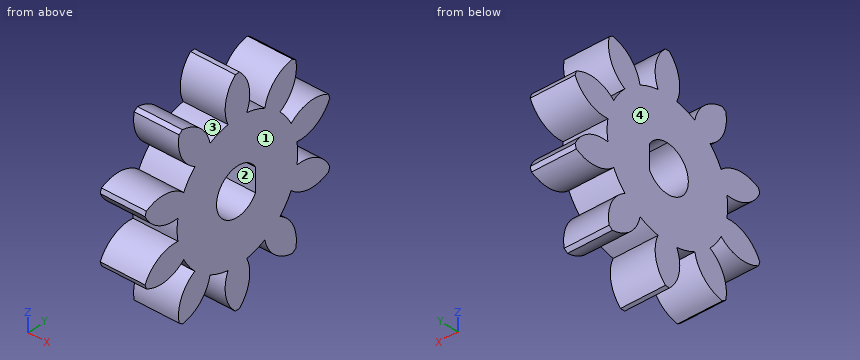
```python
from build123d import *

# Parameters (mm, degrees)
BASPROSKE_W        = 5
BASPROSKE_H        = 12
TOOTHCUT_DEPTH     = 18.691806013
TEETHCUTS_COUNT    = 10
TEETHCUTS_ANGLE    = 324
BORSKE_R           = 0.5
BORE_DEPTH         = 50.0000508
SKETCH2_R          = 0.5
CUT_EXTRUDE1_DEPTH = 10


with BuildPart() as part:
    # BasProSke → Base-Revolve (revolve)
    with BuildSketch(Plane(origin=(0, 0, 0), x_dir=(1, 0, 0), z_dir=(0, 1, 0)), mode=Mode.PRIVATE) as base_revolve_sk:
        with Locations((2.5, 6)):
            Rectangle(BASPROSKE_W, BASPROSKE_H)
    revolve(base_revolve_sk.sketch.rotate(Axis((-10, 0, 0), (1, 0, 0)), 180), axis=Axis((-10, 0, 0), (1, 0, 0)))

    # TooCutSke → ToothCut (cut, through all)
    with BuildSketch(Plane(origin=(0, 0, 0), x_dir=(0, 0, -1), z_dir=(1, 0, 0))):
        with BuildLine():
            ThreePointArc((1.173662691, 7.406586048), (0, 7.499), (-1.173662691, 7.406586048))
            ThreePointArc((-1.173662691, 7.406586048), (-1.668191438, 9.834565786), (-3.497907776, 11.50542856))
            ThreePointArc((-3.497907776, 11.50542856), (0, 12.0254), (3.497907776, 11.50542856))
            ThreePointArc((3.497907776, 11.50542856), (1.668191438, 9.834565786), (1.173662691, 7.406586048))
        make_face()
    toothcut = extrude(amount=TOOTHCUT_DEPTH, mode=Mode.SUBTRACT)

    # TeethCuts: ToothCut ×10 about axis
    teethcuts_axis = Axis((-10, 0, 0), (1, 0, 0))
    for i in range(1, TEETHCUTS_COUNT):
        add(toothcut.rotate(teethcuts_axis, i * TEETHCUTS_ANGLE / (TEETHCUTS_COUNT - 1)), mode=Mode.SUBTRACT)

    # BorSke → Bore (cut, symmetric)
    with BuildSketch(Plane(origin=(0, 0, 0), x_dir=(0, 0, -1), z_dir=(1, 0, 0))):
        with Locations(Location((0, 0, 0), (0, 0, 180))):
            Circle(BORSKE_R)
    extrude(amount=BORE_DEPTH, both=True, mode=Mode.SUBTRACT)

    # Sketch2 → Cut-Extrude1 (cut)
    with BuildSketch(Plane.ZY):
        with BuildLine():
            Line((1.302881422, 2.25), (-1.302881422, 2.25))
            ThreePointArc((-1.302881422, 2.25), (-1.29855849, -2.252497691), (2.6, 0))
            ThreePointArc((2.6, 0), (2.252497691, 1.29855849), (1.302881422, 2.25))
        make_face()
        Circle(SKETCH2_R, mode=Mode.SUBTRACT)
    extrude(amount=-CUT_EXTRUDE1_DEPTH, mode=Mode.SUBTRACT)


solid = part.part
```
Geometry check sheet. Reference: the model listing, model coordinates, mm. Face numbers are marked on the shaded views. A direction names the side the tool comes from. Coordinates: 2 decimals unless noted, no trailing zeros. Loops run counter-clockwise (first coordinate to the right, second up) from the corner with the lowest first, then second, coordinate; pieces in that order, holes last.
Item 1: Access from +Z, -Z, +X, -X, +Y, -Y to the whole of each face (thin tool, end or side, straight path). Record for the marked faces 1 and 2.
Item 2: Go/stop test with flat-tipped pins: pin 1 Ø4 at (y, z) = (0, 0) entering from -X; pin 2 Ø5 at (y, z) = (0, -6) entering from -X. Record where each tip stops, or that it passes through.
Item 3: Release check for a two-part mould opening along Y. For the marked faces 3 and 4 record: released by +Y, released by -Y, zero draft, split by the parting line, or undercut.
Item 4: Sectioned sample at D-D, the plane y = 9.75. Record the boundary of the cut face in (x, z), then the cut area to 3 significant figures.
Item 5: Thickness scan on line 1 (Z direction, x = 2.45, y = 0); line 2 (Z direction, x = 1.95, y = 6.5); line 3 (Y direction, x = 1.25, z = 0). Record the ranges inside material, lowest first.
Item 6: Sectioned sample at C-C, the plane z = -7. Record the boundary of the cut face in (x, y), then the cut area to 3 significant figures.
Item 7: Sectioned sample at B-B, the plane y = 6. Record the boundary of the cut face in (x, z).
Item 8: Sectioned sample at A-A, the plane z = 0. Record the boundary of the cut face in (x, y), then the cut area to 3 significant figures.
Check result:
1. face 1: +Z, -Z, +X, +Y, -Y
1. face 2: +X, -X
2. pin 1: passes through
2. pin 2: stops at x = 0
3. face 3: undercut
3. face 4: zero draft
4. outline: (0, -4.44) - (5, -4.44) - (5, -1.62) - (0, -1.62) - close; (0, 1.62) - (5, 1.62) - (5, 4.44) - (0, 4.44) - close
4. area: 28.2 mm2
5. line 1: z = -12 to -2.6, 2.6 to 12
5. line 2: z = -9.8 to -6.34, -3.74 to 3.74, 6.34 to 9.8
5. line 3: y = -7.5 to -2.6, 2.25 to 7.5
6. outline: (0, -6.91) - (5, -6.91) - (5, -3.48) - (0, -3.48) - close; (0, -2.69) - (5, -2.69) - (5, 2.69) - (0, 2.69) - close; (0, 3.48) - (5, 3.48) - (5, 6.91) - (0, 6.91) - close
6. area: 61.2 mm2
7. outline: (0, -9.66) - (5, -9.66) - (5, -5.8) - (0, -5.8) - close; (0, -4.5) - (5, -4.5) - (5, 4.5) - (0, 4.5) - close; (0, 5.8) - (5, 5.8) - (5, 9.66) - (0, 9.66) - close
8. outline: (0, -7.5) - (5, -7.5) - (5, -2.6) - (0, -2.6) - close; (0, 2.25) - (5, 2.25) - (5, 7.5) - (0, 7.5) - close
8. area: 50.7 mm2
